Can you work these out from the model? Positions are in its coordinate system, mm. Face numbers are marked on the shaded views. Round coordinates to 2 decimals unless told otherwise and drop trailing zeros. Loops run counter-clockwise (first coordinate to the right, second up) from the corner with the lowest first, then second, coordinate; pieces in that order, holes last. Notation, with made-up numbers: (48, 30) -> (71, 30) arc R18 cw to (71, 36) -> close; hole circle Ø4 at (75.5, 0). An arc over 180 degrees is marked (long way). Answer as a JSON object with one key per item and string values.
```python
from build123d import *

# Parameters (mm, degrees)
F0_R     = 35
F0_R_2   = 7.5
F0_R_3   = 13.5
F0_R_4   = 11
F1_DEPTH = 5
F2_DEPTH = 60


with BuildPart() as f1:
    # F0 (on Top) → F1 (new body)
    with BuildSketch(Plane.XY):
        Circle(F0_R)
        with Locations((-17.67767, -17.67767)):
            Circle(F0_R_2, mode=Mode.SUBTRACT)
        with Locations((0, -25)):
            Circle(F0_R_2, mode=Mode.SUBTRACT)
        with Locations((17.67767, -17.67767)):
            Circle(F0_R_2, mode=Mode.SUBTRACT)
        with Locations((-25, 0)):
            Circle(F0_R_2, mode=Mode.SUBTRACT)
        with Locations((-17.67767, 17.67767)):
            Circle(F0_R_2, mode=Mode.SUBTRACT)
        Circle(F0_R_3, mode=Mode.SUBTRACT)
        with Locations((25, 0)):
            Circle(F0_R_2, mode=Mode.SUBTRACT)
        with Locations((0, 25)):
            Circle(F0_R_2, mode=Mode.SUBTRACT)
        with Locations((17.67767, 17.67767)):
            Circle(F0_R_2, mode=Mode.SUBTRACT)
        Circle(F0_R_3)
        Circle(F0_R_4, mode=Mode.SUBTRACT)
        Circle(F0_R_4)
    extrude(amount=-F1_DEPTH)

    # F0 (on Top) → F2 (join)
    with BuildSketch(Plane.XY):
        Circle(F0_R_3)
        Circle(F0_R_4, mode=Mode.SUBTRACT)
    extrude(amount=F2_DEPTH)


solid = f1.part
```
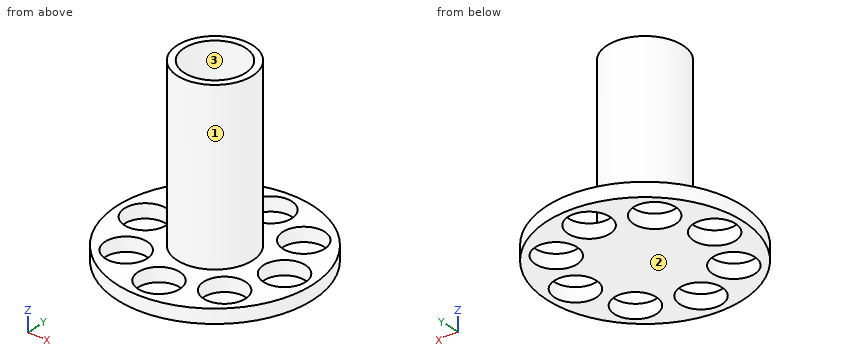
Q1. We'd pull the mould along X, two halves only. Please class the marked faces 1, 2 and 3: pulls with the +X half, pulls with the -X half, needs draft (parallel to the pull), parting line crosses it, or undercut.
Determined:
{"face 1": "parting line crosses it", "face 2": "needs draft", "face 3": "undercut"}
Q2. I want a section at B-B, the plane y = 3. Write out the boundary of the cut face in (x, z), then the cut area to 3 significant figures.
Determined:
{"outline": "(-34.87, -5) -> (-31.87, -5) -> (-31.87, 0) -> (-34.87, 0) -> close; (-18.13, -5) -> (18.13, -5) -> (18.13, 0) -> (13.16, 0) -> (13.16, 60) -> (10.58, 60) -> (10.58, 0) -> (-10.58, 0) -> (-10.58, 60) -> (-13.16, 60) -> (-13.16, 0) -> (-18.13, 0) -> close; (31.87, -5) -> (34.87, -5) -> (34.87, 0) -> (31.87, 0) -> close", "area": "521 mm²"}
Q3. I'm going to push flat-ended pins straight in: pin 1 (6 mm diameter, centred on y = 1.5, z = 19.5, fed in from -X); pin 2 (1 mm diameter, centred on x = 9.5, z = 20.5, fed in from +Y); pin 3 (6.5 mm diameter, centred on x = 2.5, y = -4, fed in from +Z). Where does each tip first touch, or does it pass through?
Determined:
{"pin 1": "x = -13.5", "pin 2": "y = 10.06", "pin 3": "z = 0"}
Q4. I want a section at D-D, the plane x = 30. Write out the boundary of the cut face in (y, z), then the cut area to 3 significant figures.
Determined:
{"outline": "(-18.03, -5) -> (-5.59, -5) -> (-5.59, 0) -> (-18.03, 0) -> close; (5.59, -5) -> (18.03, -5) -> (18.03, 0) -> (5.59, 0) -> close", "area": "124 mm²"}
Q5. If I drill on L1, parallel to Y at x = 0, z = -3.9; L2, parallel to X at y = -11, z = -2; L3, parallel to Z at x = -2, y = -1.5, over which ranges is the centre line in solid material (lowest first)? Write a range as [from, to].
Determined:
{"L1": "[-35, -32.5], [-17.5, 17.5], [32.5, 35]", "L2": "[-33.23, -21.09], [-14.26, 14.26], [21.09, 33.23]", "L3": "[-5, 0]"}
Q6. I want a section at C-C, the plane z = 7. Write out the boundary of the cut face in (x, y).
Determined:
{"outline": "circle Ø27 at (0, 0); hole circle Ø22 at (0, 0)"}
Q7. I want a section at A-A, the plane x = 0. Write out the boundary of the cut face in (y, z), then the cut area to 3 significant figures.
Determined:
{"outline": "(-35, -5) -> (-32.5, -5) -> (-32.5, 0) -> (-35, 0) -> close; (-17.5, -5) -> (17.5, -5) -> (17.5, 0) -> (13.5, 0) -> (13.5, 60) -> (11, 60) -> (11, 0) -> (-11, 0) -> (-11, 60) -> (-13.5, 60) -> (-13.5, 0) -> (-17.5, 0) -> close; (32.5, -5) -> (35, -5) -> (35, 0) -> (32.5, 0) -> close", "area": "500 mm²"}
